```python
from build123d import *

# Parameters (mm, degrees)
SKETCH1_R           = 7.5
BOSS_EXTRUDE1_DEPTH = 3
FILLET1_R           = 1
SKETCH2_W           = 1.4
SKETCH2_H           = 5.1
CUT_EXTRUDE1_DEPTH  = 2
FILLET2_R           = 0.25


with BuildPart() as part:
    # Sketch1 → Boss-Extrude1 (new body)
    with BuildSketch(Plane(origin=(0, 0, 0), x_dir=(1, 0, 0), z_dir=(0, 1, 0))):
        with Locations(Location((0, 0, 0), (0, 0, 270))):  # turned: the seam where the file's is
            Circle(SKETCH1_R)
    extrude(amount=BOSS_EXTRUDE1_DEPTH)

    # Fillet1
    fillet1_edges = [part.edges().sort_by_distance(p)[0] for p in [
        (0, 0, -7.5),
    ]]
    fillet(fillet1_edges, radius=FILLET1_R)

    # Sketch2 → Cut-Extrude1 (cut)
    with BuildSketch(Plane.XZ):
        Rectangle(SKETCH2_W, SKETCH2_H)
    extrude(amount=-CUT_EXTRUDE1_DEPTH, mode=Mode.SUBTRACT)

    # Fillet2
    fillet2_edges = [part.edges().sort_by_distance(p)[0] for p in [
        (-0.7, 0, 0),
        (0.7, 0, 0),
        (0, 3, -7.5),
    ]]
    fillet(fillet2_edges, radius=FILLET2_R)


solid = part.part
```
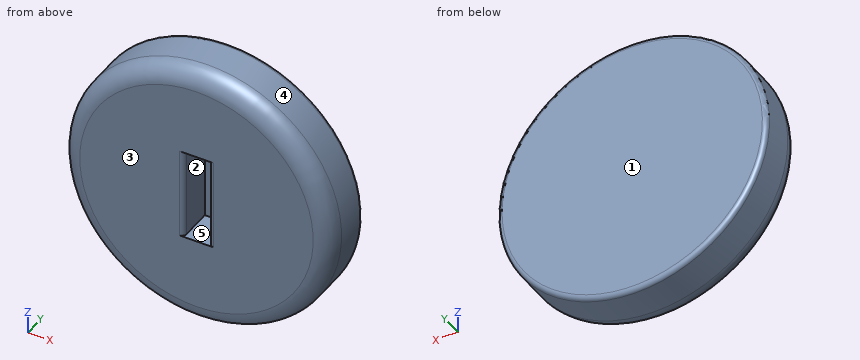
For this review, take the finished solid that the model builds, in its own axes (mm). Face numbers are marked on the shaded views. A direction names the side the tool comes from. Round coordinates to 2 decimals unless told otherwise and drop trailing zeros. Loops run counter-clockwise (first coordinate to the right, second up) from the corner with the lowest first, then second, coordinate; pieces in that order, holes last.
Q1. Add section A-A on x = 0. Write out the cut boundary in (y, z).
Result sheet:
outline: (0, -6.5) arc R1 ccw to (1, -7.5) - (2.75, -7.5) arc R0.25 ccw to (3, -7.25) - (3, 7.25) arc R0.25 ccw to (2.75, 7.5) - (1, 7.5) arc R1 ccw to (0, 6.5) - (0, 2.55) - (2, 2.55) - (2, -2.55) - (0, -2.55) - close
Q2. Add section B-B on y = 1.45. Write out the cut boundary in (x, z).
Result sheet:
outline: circle Ø15 at (0, 0); hole (-0.7, -2.55) - (0.7, -2.55) - (0.7, 2.55) - (-0.7, 2.55) - close
Q3. Machinability: for the marked faces 1 and 2, which of the approach directions +Z, -Z, +X, -X, +Y, -Y give a long, thin tool a straight path to every point of the face, cutting with its end or side? Answer none if there is none.
Result sheet:
face 1: +Z, -Z, +X, -X, +Y
face 2: -Y
Q4. Add section C-C on z = 0. Write out the cut boundary in (x, y).
Result sheet:
outline: (-7.5, 1) arc R1 ccw to (-6.5, 0) - (-0.95, 0) arc R0.25 ccw to (-0.7, 0.25) - (-0.7, 2) - (0.7, 2) - (0.7, 0.25) arc R0.25 ccw to (0.95, 0) - (6.5, 0) arc R1 ccw to (7.5, 1) - (7.5, 2.75) arc R0.25 ccw to (7.25, 3) - (-7.25, 3) arc R0.25 ccw to (-7.5, 2.75) - close
Q5. Mouldability with a two-part tool opening along Z and no side actions: class the marked faces 3, 4 and 5 as +Z half, -Z half, draft (parallel to the pull), parting line (faces both ways), or undercut.
Result sheet:
face 3: draft
face 4: parting line
face 5: undercut
Q6. Insertion check: pin 1 Ø1.5 at (y, z) = (1.5, 5) entering from +X; pin 2 Ø0.5 at (y, z) = (1, -0.5) entering from +X; pin 3 Ø1.4 at (y, z) = (1.5, -0.5) entering from -X. Each pin has a flat end and moves straight along its axis. Give the tip position at first contact, or say it passes through.
Result sheet:
pin 1: stops at x = 6.18
pin 2: stops at x = 7.5
pin 3: stops at x = -7.5
Q7. To check wall thickness, follow line 1 along X through (y, z) = (1.9, 0.25); line 2 along X through (y, z) = (0.35, -0.25); line 3 along Y through (x, z) = (6.5, -3). State the ranges of each line that lie inside material, in increasing order.
Result sheet:
line 1: x = -7.5 to -0.7, 0.7 to 7.5
line 2: x = -7.26 to -0.7, 0.7 to 7.26
line 3: y = 0.25 to 3
